from build123d import *

# Parameters (mm, degrees)
F0_W     = 31.75
F0_H     = 82.55
F1_DEPTH = 25.4
F2_W     = 31.75
F2_H     = 15.875
F3_DEPTH = 12.7
F5_D     = 3.7973
F5_DEPTH = 12.7
F5_TIP   = 1.1408240143
F7_D     = 2.7051
F7_DEPTH = 9.525
F7_TIP   = 0.8126940303


with BuildPart() as f1:
    # F0 (on Top) → F1 (new body)
    with BuildSketch(Plane.XY):
        with Locations((15.875, -41.275)):
            Rectangle(F0_W, F0_H)
    extrude(amount=F1_DEPTH)

    # F2 (on face) → F3 (cut)
    with BuildSketch(Plane(origin=(0, 0, 0), x_dir=(-1, 0, 0), z_dir=(0, 1, 0))):
        with Locations((-15.875, 17.4625)):
            Rectangle(F2_W, F2_H)
    extrude(amount=-F3_DEPTH, mode=Mode.SUBTRACT)

    # F5
    with Locations(Plane(origin=(0, 0, 0), x_dir=(-1, 0, 0), z_dir=(0, 1, 0))):
        with Locations((-25.4, 4.7752), (-6.35, 4.7752)):
            Hole(F5_D / 2, depth=F5_DEPTH)
            with Locations((0, 0, -(F5_DEPTH + F5_TIP / 2))):  # 118° drill point
                Cone(0, F5_D / 2, F5_TIP, mode=Mode.SUBTRACT)

    # F7
    with Locations(Plane.YZ.offset(31.75)):
        with Locations((-19.8374, 19.685), (-75.4126, 19.685)):
            Hole(F7_D / 2, depth=F7_DEPTH)
            with Locations((0, 0, -(F7_DEPTH + F7_TIP / 2))):  # 118° drill point
                Cone(0, F7_D / 2, F7_TIP, mode=Mode.SUBTRACT)


solid = f1.part
The listing builds one solid part. Answer for the finished solid, in the listing's coordinates (mm). A direction names the side the tool comes from. Round coordinates to 2 decimals unless told otherwise and drop trailing zeros. Order: outer loops, then holes, each group sorted by start corner. A loop starts at its lowest first (then second) coordinate and runs counter-clockwise, first axis right, second up. Notation, with made-up numbers: M 43.5,28.5 L 58.5,28.5 A17 cw 58.5,51.5 Z; hole C 86.25,1.25 d9. An arc over 180 degrees is marked long. Answer in a Markdown table with one row per item. Add a question column.
1) The part is cut by section A-A on x = 3.5. Determine the outline of the cut face in (y, z) (3 decimals).
2) Which of the six approach directions +Z, -Z, +X, -X, +Y, -Y give full straight-line access (tool end or side, diameter ignored) to faces 1 (the face through (16, -12.7, 18)), 2 (the face through (24.99, -6.44, 2.92)), 3 (the face through (26.92, -74.06, 19.74))?
3) The part is cut by section B-B on z = 14.75. Determine the outline of the cut face in (x, y).
4) Consider line 1 along Y through (x, z) = (7.5, 10); line 2 along Z through (x, y) = (6, -8) (3 decimals). Determine where each line is inside the solid, lowest interval first. Write a range as from..to.
5) Determine the mould class of faces 4 (the face through (16, -6, 9.525)), 5 (the face through (16, -41, 0)), 6 (the face through (21.553, -20.072, 19.695)) for opening direction Z: pulls with the +Z half, pulls with the -Z half, needs draft (parallel to the pull), parting line crosses it, or undercut.
6) Flat-ended cylindrical pins translate along their axes: pin 1 Ø3.5 at (x, z) = (25.4, 4.78) entering from +Y; pin 2 Ø3 at (y, z) = (-61.5, 10.5) entering from -X; pin 3 Ø6.5 at (x, y) = (16, -4) entering from +Z (3 decimals). Find the tip coordinate at first contact, or state that the pin passes through.
Findings below:
| question | item | result |
|---|---|---|
| 1 | outline | M -82.55,0 L 0,0 L 0,9.525 L -12.7,9.525 L -12.7,25.4 L -82.55,25.4 Z |
| 2 | face 1 | +Z, +X, -X, +Y |
| 2 | face 2 | +Y |
| 2 | face 3 | +X |
| 3 | outline | M 0,-82.55 L 31.75,-82.55 L 31.75,-12.7 L 0,-12.7 Z |
| 4 | line 1 | y = -82.55..-12.7 |
| 4 | line 2 | z = 0..2.909, 6.641..9.525 |
| 5 | face 4 | pulls with the +Z half |
| 5 | face 5 | pulls with the -Z half |
| 5 | face 6 | undercut |
| 6 | pin 1 | stops at y = -12.79 |
| 6 | pin 2 | stops at x = 0 |
| 6 | pin 3 | stops at z = 9.525 |
